Study the drawing (mm; zero at the part's minimum x, y, z) and answer. A direction names the side the tool comes from. Coordinates: 2 decimals unless noted, no trailing zeros. Write each loop counter-clockwise with the first axis right and the second up, starting at its lowest first coordinate (ties: lowest second). Pieces come first, ordered by that corner, then holes. Notation, with made-up numbers: (-16.75, 48) -> (30.25, 48) arc R29 cw to (30.25, 87) -> close; hole circle Ø11 at (59, 57). An arc over 180 degrees is marked (long way). Answer in a Markdown table with one row per item. Add a question column.
Item 1: Section C-C on x = 40 is taken. Write down the section's boundary in (y, z), then the cut area to 3 significant figures.
Item 2: Section B-B on y = 32.5 is taken. Write down the section's boundary in (x, z).
Item 3: Given pin 1 Ø5 at (x, z) = (37.5, 9.5) entering from -Y; pin 2 Ø3 at (x, y) = (24, 10.5) entering from -Z, each flat-ended and moving along its own axis, determine where each tip first touches the part or whether it passes through.
Item 4: Section A-A on z = 10.5 is taken. Write down the section's boundary in (x, y).
Item 5: For a pull along X with two mould halves and no side action, classify the marked faces 1, 2, 3 and 4 as +X half, -X half, draft (parallel to the pull), parting line (faces both ways), or undercut.
Item 6: Which of the six approach directions +Z, -Z, +X, -X, +Y, -Y give full straight-line access (tool end or side, diameter ignored) to the marked faces 5 and 6?
Item 7: Straight lines are drawn through the part: line 1 (X direction, y = 23, z = 5.25); line 2 (Y direction, x = 10, z = 16); line 3 (Z direction, x = 66, y = 67). For each, find the intervals that lie inside material, in ascending order. Write a range as from..to.
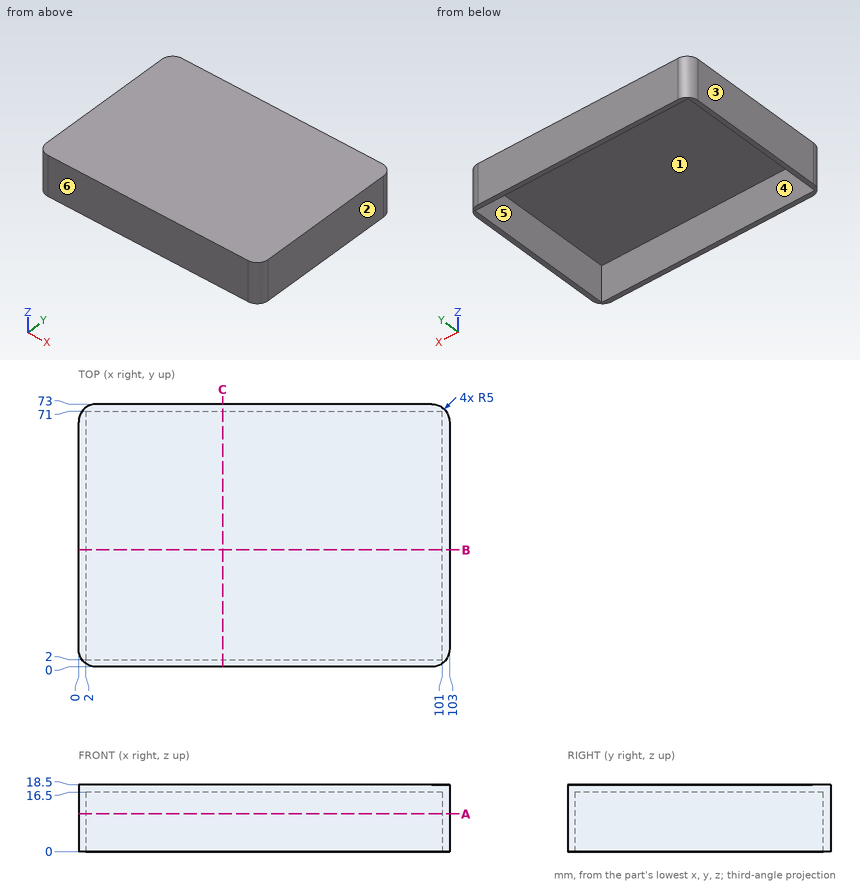
Results below:
| question | item | result |
|---|---|---|
| 1 | outline | (0, 0) -> (2, 0) -> (2, 16.5) -> (71, 16.5) -> (71, 0) -> (73, 0) -> (73, 18.5) -> (0, 18.5) -> close |
| 1 | area | 212 mm2 |
| 2 | outline | (0, 0) -> (2, 0) -> (2, 16.5) -> (101, 16.5) -> (101, 0) -> (103, 0) -> (103, 18.5) -> (0, 18.5) -> close |
| 3 | pin 1 | stops at y = 0 |
| 3 | pin 2 | stops at z = 16.5 |
| 4 | outline | (0, 5) arc R5 ccw to (5, 0) -> (98, 0) arc R5 ccw to (103, 5) -> (103, 68) arc R5 ccw to (98, 73) -> (5, 73) arc R5 ccw to (0, 68) -> close; hole (2, 2) -> (101, 2) -> (101, 71) -> (2, 71) -> close |
| 5 | face 1 | undercut |
| 5 | face 2 | +X half |
| 5 | face 3 | -X half |
| 5 | face 4 | undercut |
| 6 | face 5 | -Z |
| 6 | face 6 | +Z, -Z, +X, -X, -Y |
| 7 | line 1 | x = 0..2, 101..103 |
| 7 | line 2 | y = 0..2, 71..73 |
| 7 | line 3 | z = 16.5..18.5 |
